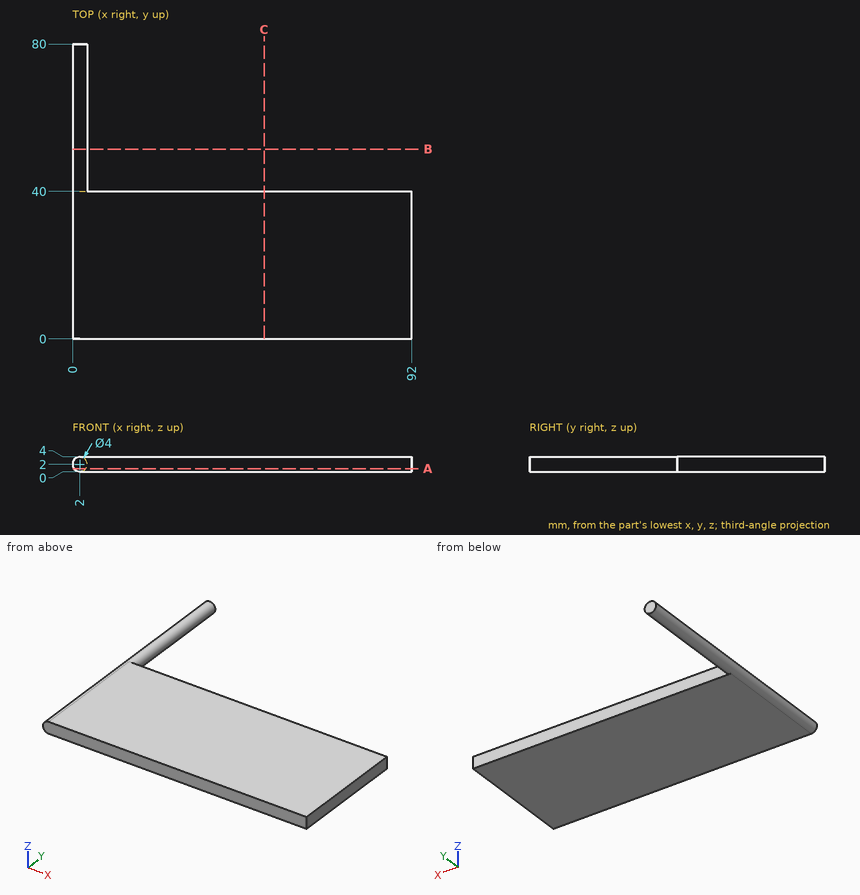
Part print with two shaded views. Sizes in mm from the minimum x, y, z corner. Give positions to 0.01 mm unless a question says otherwise; leave off trailing zeros. Order: outer loops, then holes, each group sorted by start corner. A loop starts at its lowest first (then second) coordinate and runs counter-clockwise, first axis right, second up.
1) Saw through at C-C, the plane x = 52. Write the cut outline in (y, z), then the cut area to 3 significant figures.
2) Wall check: probe 1 along Y at (x, z) = (26.5, 0.35); probe 2 along X at (y, z) = (28, 1.85); probe 3 along X at (y, z) = (13, 3.6). Give the ranges that are in metal, low to high.
3) Saw through at A-A, the plane z = 0.8. Write the cut outline in (x, y), then the cut area to 3 significant figures.
4) Saw through at B-B, the plane y = 51.5. Write the cut outline in (x, z).
5) Pin check, flat tips, straight feed: pin 1 (1.5 mm diameter, centred on x = 52, z = 3.5, fed in from +Y); pin 2 (6 mm diameter, centred on x = 69.5, y = 30.5, fed in from -Z). Stop position of each tip, or through.
Computed:
1. outline: (0, 0) - (40, 0) - (40, 4) - (0, 4) - close
1. area: 160 mm2
2. probe 1: y = 0 to 40
2. probe 2: x = 0.01 to 92
2. probe 3: x = 0.8 to 92
3. outline: (0.4, 0) - (92, 0) - (92, 40) - (3.6, 40) - (3.6, 80) - (0.4, 80) - close
3. area: 3,790 mm2
4. outline: circle Ø4 at (2, 2)
5. pin 1: stops at y = 40
5. pin 2: stops at z = 0
